Source: three-view drawing plus pictorial views. Frame: mm from the lowest corner of the part. A direction names the side the tool comes from. Round coordinates to 2 decimals unless told otherwise and drop trailing zeros. Write each loop counter-clockwise with the first axis right and the second up, starting at its lowest first coordinate (ties: lowest second). Pieces come first, ordered by that corner, then holes. Notation, with made-up numbers: M 60.5,28 L 99.5,28 A30 cw 99.5,58 Z; hole C 87,51.25 d2. An arc over 180 degrees is marked long. Answer as CSV lines item,"result". Start each with the question number.
Q1. Mould query, pull axis Y, two halves, no side actions, for the marked faces 3, 4 and 5. Classes: pulls with the +Y half, pulls with the -Y half, needs draft (parallel to the pull), parting line crosses it, or undercut.
Q2. First-contact query: pin 1 (6 mm diameter, centred on y = 508, z = 38.5, fed in from -X); pin 2 (11.5 mm diameter, centred on y = 138.5, z = 24.5, fed in from +X); pin 3 (13 mm diameter, centred on x = 25.5, y = 634.5, fed in from -Z); pin 4 (8 mm diameter, centred on y = 635.5, z = 26.5, fed in from -X). Flat tips, straight axial feed; report the tip coordinate or a pass-through.
Q3. Reachability of the marked faces 1 and 2 from +Z, -Z, +X, -X, +Y, -Y: full face, straight path, thin tool, end or side. Return the list, or none.
Q4. Section query C-C on x = 25.4. Output: boundary loops of the cut face in (y, z).
Q5. Section query B-B on y = 25.4. Output: boundary loops of the cut face in (x, z), and give its area (3 significant figures).
Q6. Section query A-A on z = 5.5. Output: boundary loops of the cut face in (x, y), and give its area (3 significant figures).
Q7. Ray query, probe 1 along Y at (x, z) = (25.4, 11.5); probe 2 along X at (y, z) = (635, 7.75); probe 3 along Z at (x, y) = (4, 25). Return the intervals inside material, ascending.
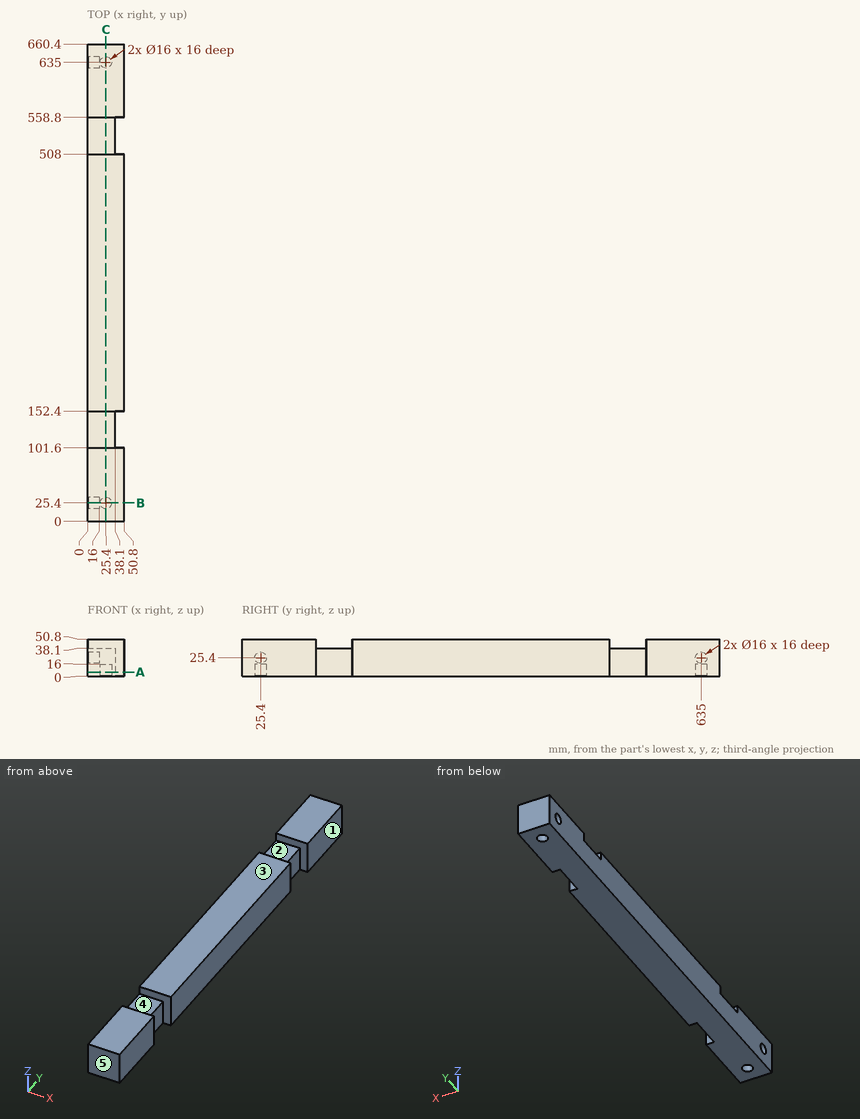
Entries:
1,face 3,"needs draft"
1,face 4,"undercut"
1,face 5,"pulls with the -Y half"
2,pin 1,"stops at x = 0"
2,pin 2,"stops at x = 38.1"
2,pin 3,"stops at z = 16"
2,pin 4,"stops at x = 16"
3,face 1,"+Z, -Z, +X, +Y, -Y"
3,face 2,"+Z, +X, -X"
4,outline,"M 0,0 L 17.4,0 L 17.4,16 L 33.4,16 L 33.4,0 L 627,0 L 627,16 L 643,16 L 643,0 L 660.4,0 L 660.4,50.8 L 558.8,50.8 L 558.8,38.1 L 508,38.1 L 508,50.8 L 152.4,50.8 L 152.4,38.1 L 101.6,38.1 L 101.6,50.8 L 0,50.8 Z"
5,outline,"M 0,0 L 17.4,0 L 17.4,16 L 33.4,16 L 33.4,0 L 50.8,0 L 50.8,50.8 L 0,50.8 L 0,33.4 L 16,33.4 L 16,17.4 L 0,17.4 Z"
5,area,"2,070 mm^2"
6,outline,"M 0,0 L 50.8,0 L 50.8,101.6 L 38.1,101.6 L 38.1,152.4 L 50.8,152.4 L 50.8,508 L 38.1,508 L 38.1,558.8 L 50.8,558.8 L 50.8,660.4 L 0,660.4 Z; hole C 25.4,25.4 d16; hole C 25.4,635 d16"
6,area,"31,900 mm^2"
7,probe 1,"y = 0 to 17.4, 33.4 to 627, 643 to 660.4"
7,probe 2,"x = 0 to 17.4, 33.4 to 50.8"
7,probe 3,"z = 0 to 17.41, 33.39 to 50.8"
